Source: three-view drawing plus pictorial views. Frame: mm from the lowest corner of the part. Give positions to 0.01 mm unless a question says otherwise; leave off trailing zeros. Loops run counter-clockwise (first coordinate to the right, second up) from the corner with the lowest first, then second, coordinate; pieces in that order, holes last.
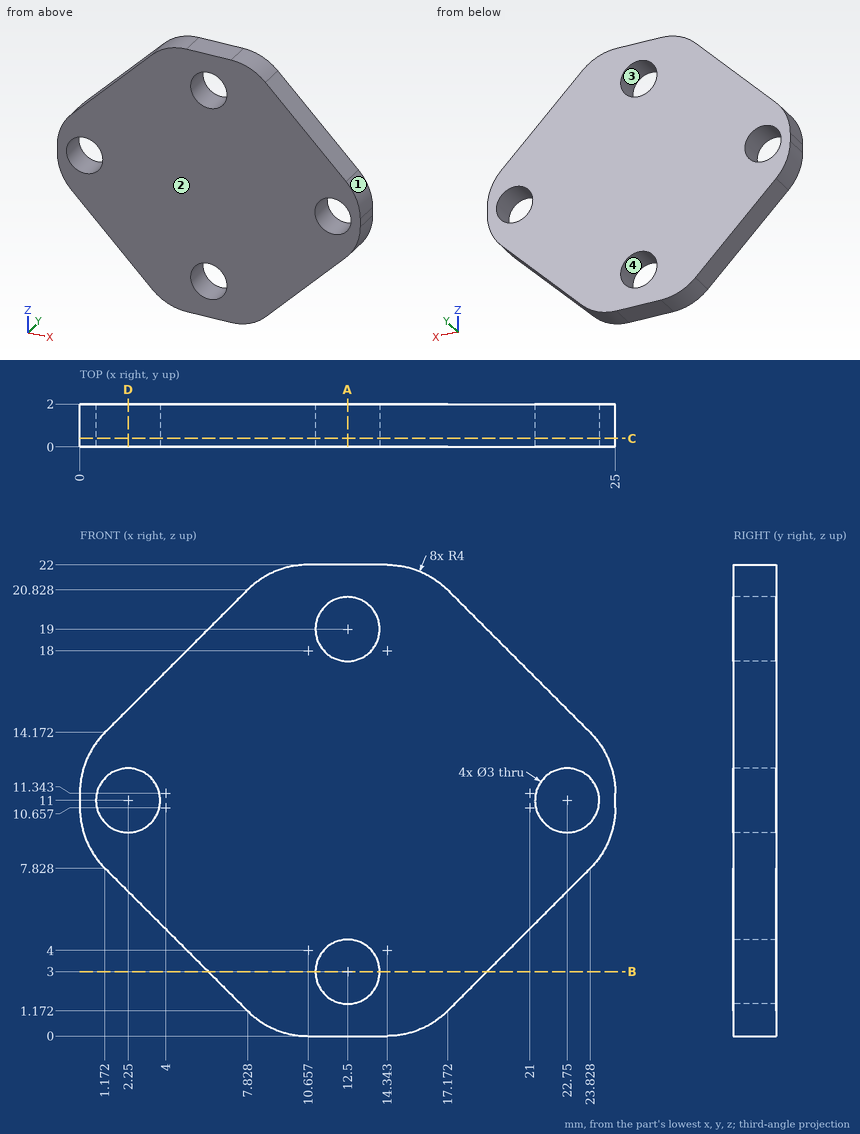
Q1. Section query A-A, the plane x = 12.5. Return loops of the section in (y, z).
Q2. Pin query (flat end, axial travel): pin 1 Ø5 at (x, z) = (12.5, 19) entering from -Y; pin 2 Ø1 at (y, z) = (1.5, 8.5) entering from +X. Return the tip coordinate at first contact, or that it passes through.
Q3. Material intervals for probe 1 along Z at (x, y) = (12.5, 1.1); probe 2 along X at (y, z) = (1.35, 11); probe 3 along Z at (x, y) = (22.75, 1.5), sorted ascending.
Q4. Section query D-D, the plane x = 2.25. Return loops of the section in (y, z).
Q5. Mould query, pull axis X, two halves, no side actions, for the marked faces 1, 2, 3 and 4. Classes: +X half, -X half, draft (parallel to the pull), parting line (faces both ways), or undercut.
Q6. Section query B-B, the plane z = 3. Return loops of the section in (x, y), and give its area (3 significant figures).
Q7. Section query C-C, the plane y = 0.4. Return loops of the section in (x, z), and give its area (3 significant figures).
Resolved:
1. outline: (0, 0) - (2, 0) - (2, 1.5) - (0, 1.5) - close; (0, 4.5) - (2, 4.5) - (2, 17.5) - (0, 17.5) - close; (0, 20.5) - (2, 20.5) - (2, 22) - (0, 22) - close
2. pin 1: stops at y = 0
2. pin 2: stops at x = 24.64
3. probe 1: z = 0 to 1.5, 4.5 to 17.5, 20.5 to 22
3. probe 2: x = 0 to 0.75, 3.75 to 21.25, 24.25 to 25
3. probe 3: z = 6.75 to 9.5, 12.5 to 15.25
4. outline: (0, 6.75) - (2, 6.75) - (2, 9.5) - (0, 9.5) - close; (0, 12.5) - (2, 12.5) - (2, 15.25) - (0, 15.25) - close
5. face 1: +X half
5. face 2: draft
5. face 3: undercut
5. face 4: undercut
6. outline: (6, 0) - (11, 0) - (11, 2) - (6, 2) - close; (14, 0) - (19, 0) - (19, 2) - (14, 2) - close
6. area: 20.0 mm2
7. outline: (0, 10.66) arc R4 ccw to (1.17, 7.83) - (7.83, 1.17) arc R4 ccw to (10.66, 0) - (14.34, 0) arc R4 ccw to (17.17, 1.17) - (23.83, 7.83) arc R4 ccw to (25, 10.66) - (25, 11.34) arc R4 ccw to (23.83, 14.17) - (17.17, 20.83) arc R4 ccw to (14.34, 22) - (10.66, 22) arc R4 ccw to (7.83, 20.83) - (1.17, 14.17) arc R4 ccw to (0, 11.34) - close; hole circle Ø3 at (2.25, 11); hole circle Ø3 at (12.5, 3); hole circle Ø3 at (12.5, 19); hole circle Ø3 at (22.75, 11)
7. area: 357 mm2
